Model file for the job. Use its own axes, mm. Face numbers are marked on the shaded views. A direction names the side the tool comes from. Coordinates: 2 decimals unless noted, no trailing zeros. Write each loop counter-clockwise with the first axis right and the second up, starting at its lowest first coordinate (ties: lowest second). Pieces come first, ordered by that corner, then holes.
Q1. Pin check, flat tips, straight feed: P1, Ø0.9, axis at y = 295.5, z = 2, coming from the -X side; P2, Ø1.5, axis at y = 315, z = 1, coming from the +X side; P3, Ø7, axis at y = 453, z = -5, coming from the +X side; P4, Ø3.5, axis at x = 91, z = 2, coming from the +Y side. Stop position of each tip, or through.
Q2. Band-saw the part on A-A, the plane z = -7.5. Write the cut outline in (x, y), plus the area to 3 significant figures.
Q3. Which spindle directions (+Z, -Z, +X, -X, +Y, -Y) get a long thin tool onto all of the face, cutting with end or side? Do the marked faces 1 and 2. Say none if no direction does.
Q4. Band-saw the part on C-C, the plane y = 223. Write the cut outline in (x, z), plus the area to 3 significant figures.
Q5. Drill centre lines: probe 1 along Y at (x, z) = (28, -5); probe 2 along X at (y, z) = (1.85, -15); probe 3 along Y at (x, z) = (-171.5, -24). Where is each one in solid material? Low to high.
Q6. Band-saw the part on B-B, the plane y = 420. Write the cut outline in (x, z).
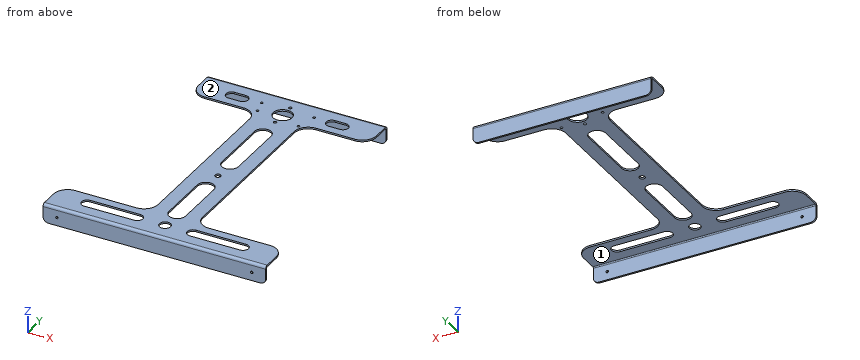
from build123d import *

# Parameters (mm, degrees)
ESQUISSE1_W                             = 400
ESQUISSE1_H                             = 470
BOSS_EXTRU_1_DEPTH                      = 3
T_LE_PLI_E_SUR_AR_TE1_STRIP_W           = 16
T_LE_PLI_E_SUR_AR_TE1_STRIP_H           = 3
T_LE_PLI_E_SUR_AR_TE1_STRIP_CUT_DEPTH   = 400
T_LE_PLI_E_SUR_AR_TE1_STRIP_2_W         = 16
T_LE_PLI_E_SUR_AR_TE1_STRIP_2_H         = 3
T_LE_PLI_E_SUR_AR_TE1_STRIP_CUT_2_DEPTH = 400
T_LE_PLI_E_SUR_AR_TE1_DEPTH             = 400
T_LE_PLI_E_SUR_AR_TE1_BEND_DEPTH        = 400
ENL_V_MAT_EXTRU_1_REACH                 = 513.849
ESQUISSE7_R                             = 17
ESQUISSE7_R_2                           = 5.1
ESQUISSE7_R_3                           = 2.75
ENL_V_MAT_EXTRU_2_REACH                 = 513.849
ESQUISSE12_R                            = 2.25
ESQUISSE12_R_2                          = 10
CONG_10_R                               = 10
CONG_2_R                                = 25
ESQUISSE13_R                            = 2.25
ENL_V_MAT_EXTRU_3_DEPTH                 = 10


# Sheet-metal steps are written as plain solids
with BuildPart() as part:
    # Esquisse1 → Boss.-Extru.1 (new body)
    with BuildSketch(Plane.XY):
        with Locations((0, 235)):
            Rectangle(ESQUISSE1_W, ESQUISSE1_H)
    extrude(amount=BOSS_EXTRU_1_DEPTH)

    # Tôle pliée sur arête1 strip (across the edge) → Tôle pliée sur arête1 strip cut (cut)
    with BuildSketch(Plane(origin=(-200, 470, 0), x_dir=(0, -1, 0), z_dir=(1, 0, 0))):
        with Locations((-3, -1.5)):
            Rectangle(T_LE_PLI_E_SUR_AR_TE1_STRIP_W, T_LE_PLI_E_SUR_AR_TE1_STRIP_H)
    extrude(amount=T_LE_PLI_E_SUR_AR_TE1_STRIP_CUT_DEPTH, mode=Mode.SUBTRACT)

    # Tôle pliée sur arête1 strip 2 (across the edge) → Tôle pliée sur arête1 strip cut 2 (cut)
    with BuildSketch(Plane(origin=(200, 0, 0), x_dir=(0, 1, 0), z_dir=(-1, 0, 0))):
        with Locations((-3, -1.5)):
            Rectangle(T_LE_PLI_E_SUR_AR_TE1_STRIP_2_W, T_LE_PLI_E_SUR_AR_TE1_STRIP_2_H)
    extrude(amount=T_LE_PLI_E_SUR_AR_TE1_STRIP_CUT_2_DEPTH, mode=Mode.SUBTRACT)

    # Tôle pliée sur arête1 section (across the edge) → Tôle pliée sur arête1 (add)
    with BuildSketch(Plane(origin=(-200, 470, 0), x_dir=(0, -1, 0), z_dir=(1, 0, 0))):
        with BuildLine():
            Line((0, 2), (0, 30))
            Line((0, 30), (3, 30))
            Line((3, 30), (3, 2))
            ThreePointArc((3, 2), (3.585786438, 0.585786438), (5, 0))
            Line((5, 0), (5, -3))
            ThreePointArc((5, -3), (1.464466094, -1.535533906), (0, 2))
        make_face()
    extrude(amount=T_LE_PLI_E_SUR_AR_TE1_DEPTH)

    # Tôle pliée sur arête1 section 2 (across the edge) → Tôle pliée sur arête1 bend (add)
    with BuildSketch(Plane(origin=(200, 0, 0), x_dir=(0, 1, 0), z_dir=(-1, 0, 0))):
        with BuildLine():
            Line((0, 2), (0, 30))
            Line((0, 30), (3, 30))
            Line((3, 30), (3, 2))
            ThreePointArc((3, 2), (3.585786438, 0.585786438), (5, 0))
            Line((5, 0), (5, -3))
            ThreePointArc((5, -3), (1.464466094, -1.535533906), (0, 2))
        make_face()
    extrude(amount=T_LE_PLI_E_SUR_AR_TE1_BEND_DEPTH)

    # Esquisse7 → Enlèv. mat.-Extru.1 (cut, up to next)
    with BuildSketch(Plane.XY.offset(3), mode=Mode.PRIVATE) as enl_v_mat_extru_1_sk1:
        with Locations((0, 420)):
            Circle(ESQUISSE7_R)
    enl_v_mat_extru_1_tool1 = extrude(enl_v_mat_extru_1_sk1.sketch, amount=-ENL_V_MAT_EXTRU_1_REACH, mode=Mode.PRIVATE) & part.part
    # Esquisse7 → Enlèv. mat.-Extru.1 (cut, up to next)
    with BuildSketch(Plane.XY.offset(3), mode=Mode.PRIVATE) as enl_v_mat_extru_1_sk2:
        with Locations((0, 208)):
            Circle(ESQUISSE7_R_2)
    enl_v_mat_extru_1_tool2 = extrude(enl_v_mat_extru_1_sk2.sketch, amount=-ENL_V_MAT_EXTRU_1_REACH, mode=Mode.PRIVATE) & part.part
    # Esquisse7 → Enlèv. mat.-Extru.1 (cut, up to next)
    with BuildSketch(Plane.XY.offset(3), mode=Mode.PRIVATE) as enl_v_mat_extru_1_sk3:
        with Locations((0, 395)):
            Circle(ESQUISSE7_R_3)
    enl_v_mat_extru_1_tool3 = extrude(enl_v_mat_extru_1_sk3.sketch, amount=-ENL_V_MAT_EXTRU_1_REACH, mode=Mode.PRIVATE) & part.part
    # Esquisse7 → Enlèv. mat.-Extru.1 (cut, up to next)
    with BuildSketch(Plane.XY.offset(3), mode=Mode.PRIVATE) as enl_v_mat_extru_1_sk4:
        with Locations((0, 445)):
            Circle(ESQUISSE7_R_3)
    enl_v_mat_extru_1_tool4 = extrude(enl_v_mat_extru_1_sk4.sketch, amount=-ENL_V_MAT_EXTRU_1_REACH, mode=Mode.PRIVATE) & part.part
    # Esquisse7 → Enlèv. mat.-Extru.1 (cut, up to next)
    with BuildSketch(Plane.XY.offset(3), mode=Mode.PRIVATE) as enl_v_mat_extru_1_sk5:
        with BuildLine():
            Line((-200, 60), (-65, 60))
            ThreePointArc((-65, 60), (-47.32233047, 67.32233047), (-40, 85))
            Line((-40, 85), (-40, 385))
            ThreePointArc((-40, 385), (-47.32233047, 402.67766953), (-65, 410))
            Line((-65, 410), (-160, 410))
            Line((-160, 410), (-160, 470))
            Line((-160, 470), (-200, 470))
            Line((-200, 470), (-200, 60))
        make_face()
    enl_v_mat_extru_1_tool5 = extrude(enl_v_mat_extru_1_sk5.sketch, amount=-ENL_V_MAT_EXTRU_1_REACH, mode=Mode.PRIVATE) & part.part
    # Esquisse7 → Enlèv. mat.-Extru.1 (cut, up to next)
    with BuildSketch(Plane.XY.offset(3), mode=Mode.PRIVATE) as enl_v_mat_extru_1_sk6:
        with BuildLine():
            Line((200.093993977, 470), (200.093993977, 60))
            Line((200.093993977, 60), (65, 60))
            ThreePointArc((65, 60), (47.32233047, 67.32233047), (40, 85))
            Line((40, 85), (40, 385))
            ThreePointArc((40, 385), (47.32233047, 402.67766953), (65, 410))
            Line((65, 410), (160, 410))
            Line((160, 410), (160, 470))
            Line((160, 470), (200.093993977, 470))
        make_face()
    enl_v_mat_extru_1_tool6 = extrude(enl_v_mat_extru_1_sk6.sketch, amount=-ENL_V_MAT_EXTRU_1_REACH, mode=Mode.PRIVATE) & part.part
    add(enl_v_mat_extru_1_tool1.solids().sort_by_distance((0, 420, 3))[0], mode=Mode.SUBTRACT)
    add(enl_v_mat_extru_1_tool2.solids().sort_by_distance((0, 208, 3))[0], mode=Mode.SUBTRACT)
    add(enl_v_mat_extru_1_tool3.solids().sort_by_distance((0, 395, 3))[0], mode=Mode.SUBTRACT)
    add(enl_v_mat_extru_1_tool4.solids().sort_by_distance((0, 445, 3))[0], mode=Mode.SUBTRACT)
    add(enl_v_mat_extru_1_tool5.solids().sort_by_distance((-122.820528, 243.463534, 3))[0], mode=Mode.SUBTRACT)
    add(enl_v_mat_extru_1_tool6.solids().sort_by_distance((122.87169, 243.477801, 3))[0], mode=Mode.SUBTRACT)

    # Esquisse12 → Enlèv. mat.-Extru.2 (cut, up to next)
    with BuildSketch(Plane.XY.offset(3), mode=Mode.PRIVATE) as enl_v_mat_extru_2_sk1:
        with Locations((38.064927056, 402.250033007)):
            Circle(ESQUISSE12_R)
    enl_v_mat_extru_2_tool1 = extrude(enl_v_mat_extru_2_sk1.sketch, amount=-ENL_V_MAT_EXTRU_2_REACH, mode=Mode.PRIVATE) & part.part
    # Esquisse12 → Enlèv. mat.-Extru.2 (cut, up to next)
    with BuildSketch(Plane.XY.offset(3), mode=Mode.PRIVATE) as enl_v_mat_extru_2_sk2:
        with Locations((-41.361925627, 412.706776538)):
            Circle(ESQUISSE12_R)
    enl_v_mat_extru_2_tool2 = extrude(enl_v_mat_extru_2_sk2.sketch, amount=-ENL_V_MAT_EXTRU_2_REACH, mode=Mode.PRIVATE) & part.part
    # Esquisse12 → Enlèv. mat.-Extru.2 (cut, up to next)
    with BuildSketch(Plane.XY.offset(3), mode=Mode.PRIVATE) as enl_v_mat_extru_2_sk3:
        with Locations((46.984631039, 437.101007166)):
            Circle(ESQUISSE12_R)
    enl_v_mat_extru_2_tool3 = extrude(enl_v_mat_extru_2_sk3.sketch, amount=-ENL_V_MAT_EXTRU_2_REACH, mode=Mode.PRIVATE) & part.part
    # Esquisse12 → Enlèv. mat.-Extru.2 (cut, up to next)
    with BuildSketch(Plane.XY.offset(3), mode=Mode.PRIVATE) as enl_v_mat_extru_2_sk4:
        with Locations((-46.984631039, 437.101007166)):
            Circle(ESQUISSE12_R)
    enl_v_mat_extru_2_tool4 = extrude(enl_v_mat_extru_2_sk4.sketch, amount=-ENL_V_MAT_EXTRU_2_REACH, mode=Mode.PRIVATE) & part.part
    # Esquisse12 → Enlèv. mat.-Extru.2 (cut, up to next)
    with BuildSketch(Plane.XY.offset(3), mode=Mode.PRIVATE) as enl_v_mat_extru_2_sk5:
        with Locations((0, 35)):
            Circle(ESQUISSE12_R_2)
    enl_v_mat_extru_2_tool5 = extrude(enl_v_mat_extru_2_sk5.sketch, amount=-ENL_V_MAT_EXTRU_2_REACH, mode=Mode.PRIVATE) & part.part
    # Esquisse12 → Enlèv. mat.-Extru.2 (cut, up to next)
    with BuildSketch(Plane.XY.offset(3), mode=Mode.PRIVATE) as enl_v_mat_extru_2_sk6:
        with BuildLine():
            Line((-15, 168), (-15, 75))
            ThreePointArc((-15, 75), (0, 60), (15, 75))
            Line((15, 75), (15, 168))
            ThreePointArc((15, 168), (0, 183), (-15, 168))
        make_face()
    enl_v_mat_extru_2_tool6 = extrude(enl_v_mat_extru_2_sk6.sketch, amount=-ENL_V_MAT_EXTRU_2_REACH, mode=Mode.PRIVATE) & part.part
    # Esquisse12 → Enlèv. mat.-Extru.2 (cut, up to next)
    with BuildSketch(Plane.XY.offset(3), mode=Mode.PRIVATE) as enl_v_mat_extru_2_sk7:
        with BuildLine():
            Line((140, 45), (50, 45))
            ThreePointArc((50, 45), (40, 35), (50, 25))
            Line((50, 25), (140, 25))
            ThreePointArc((140, 25), (150, 35), (140, 45))
        make_face()
    enl_v_mat_extru_2_tool7 = extrude(enl_v_mat_extru_2_sk7.sketch, amount=-ENL_V_MAT_EXTRU_2_REACH, mode=Mode.PRIVATE) & part.part
    # Esquisse12 → Enlèv. mat.-Extru.2 (cut, up to next)
    with BuildSketch(Plane.XY.offset(3), mode=Mode.PRIVATE) as enl_v_mat_extru_2_sk8:
        with BuildLine():
            Line((15, 355), (15, 248))
            ThreePointArc((15, 248), (0, 233), (-15, 248))
            Line((-15, 248), (-15, 355))
            ThreePointArc((-15, 355), (0, 370), (15, 355))
        make_face()
    enl_v_mat_extru_2_tool8 = extrude(enl_v_mat_extru_2_sk8.sketch, amount=-ENL_V_MAT_EXTRU_2_REACH, mode=Mode.PRIVATE) & part.part
    # Esquisse12 → Enlèv. mat.-Extru.2 (cut, up to next)
    with BuildSketch(Plane.XY.offset(3), mode=Mode.PRIVATE) as enl_v_mat_extru_2_sk9:
        with BuildLine():
            Line((-140, 45), (-50, 45))
            ThreePointArc((-50, 45), (-40, 35), (-50, 25))
            Line((-50, 25), (-140, 25))
            ThreePointArc((-140, 25), (-150, 35), (-140, 45))
        make_face()
    enl_v_mat_extru_2_tool9 = extrude(enl_v_mat_extru_2_sk9.sketch, amount=-ENL_V_MAT_EXTRU_2_REACH, mode=Mode.PRIVATE) & part.part
    # Esquisse12 → Enlèv. mat.-Extru.2 (cut, up to next)
    with BuildSketch(Plane.XY.offset(3), mode=Mode.PRIVATE) as enl_v_mat_extru_2_sk10:
        with BuildLine():
            Line((-100, 425), (-80, 425))
            ThreePointArc((-80, 425), (-70, 435), (-80, 445))
            Line((-80, 445), (-100, 445))
            ThreePointArc((-100, 445), (-110, 435), (-100, 425))
        make_face()
    enl_v_mat_extru_2_tool10 = extrude(enl_v_mat_extru_2_sk10.sketch, amount=-ENL_V_MAT_EXTRU_2_REACH, mode=Mode.PRIVATE) & part.part
    # Esquisse12 → Enlèv. mat.-Extru.2 (cut, up to next)
    with BuildSketch(Plane.XY.offset(3), mode=Mode.PRIVATE) as enl_v_mat_extru_2_sk11:
        with BuildLine():
            Line((80, 445), (100, 445))
            ThreePointArc((100, 445), (110, 435), (100, 425))
            Line((100, 425), (80, 425))
            ThreePointArc((80, 425), (70, 435), (80, 445))
        make_face()
    enl_v_mat_extru_2_tool11 = extrude(enl_v_mat_extru_2_sk11.sketch, amount=-ENL_V_MAT_EXTRU_2_REACH, mode=Mode.PRIVATE) & part.part
    add(enl_v_mat_extru_2_tool1.solids().sort_by_distance((38.064927, 402.250033, 3))[0], mode=Mode.SUBTRACT)
    add(enl_v_mat_extru_2_tool2.solids().sort_by_distance((-41.361926, 412.706777, 3))[0], mode=Mode.SUBTRACT)
    add(enl_v_mat_extru_2_tool3.solids().sort_by_distance((46.984631, 437.101007, 3))[0], mode=Mode.SUBTRACT)
    add(enl_v_mat_extru_2_tool4.solids().sort_by_distance((-46.984631, 437.101007, 3))[0], mode=Mode.SUBTRACT)
    add(enl_v_mat_extru_2_tool5.solids().sort_by_distance((0, 35, 3))[0], mode=Mode.SUBTRACT)
    add(enl_v_mat_extru_2_tool6.solids().sort_by_distance((0, 121.5, 3))[0], mode=Mode.SUBTRACT)
    add(enl_v_mat_extru_2_tool7.solids().sort_by_distance((95, 35, 3))[0], mode=Mode.SUBTRACT)
    add(enl_v_mat_extru_2_tool8.solids().sort_by_distance((0, 301.5, 3))[0], mode=Mode.SUBTRACT)
    add(enl_v_mat_extru_2_tool9.solids().sort_by_distance((-95, 35, 3))[0], mode=Mode.SUBTRACT)
    add(enl_v_mat_extru_2_tool10.solids().sort_by_distance((-90, 435, 3))[0], mode=Mode.SUBTRACT)
    add(enl_v_mat_extru_2_tool11.solids().sort_by_distance((90, 435, 3))[0], mode=Mode.SUBTRACT)

    # Congé 10
    cong_10_edges = [part.edges().sort_by_distance(p)[0] for p in [
        (160, 468.5, -30),
        (200, 1.5, -30),
        (-200, 1.5, -30),
        (-160, 468.5, -30),
    ]]
    fillet(cong_10_edges, radius=CONG_10_R)

    # Congé2
    cong_2_edges = [part.edges().sort_by_distance(p)[0] for p in [
        (200, 60, 1.5),
        (160, 410, 1.5),
        (-200, 60, 1.5),
        (-160, 410, 1.5),
    ]]
    fillet(cong_2_edges, radius=CONG_2_R)

    # Esquisse13 → Enlèv. mat.-Extru.3 (cut)
    with BuildSketch(Plane(origin=(0, 0, 0), x_dir=(-1, 0, 0), z_dir=(0, -1, 0))):
        with Locations(Location((175, 15, 0), (0, 0, 90))):
            Circle(ESQUISSE13_R)
        with Locations(Location((-175, 15, 0), (0, 0, 90))):
            Circle(ESQUISSE13_R)
    extrude(amount=-ENL_V_MAT_EXTRU_3_DEPTH, mode=Mode.SUBTRACT)


solid = part.part
Answer sheet:
1. P1: stops at x = -40
1. P2: stops at x = 40
1. P3: passes through
1. P4: stops at y = 469.47
2. outline: (-200, 0) - (200, 0) - (200, 3) - (-200, 3) - close; (-160, 467) - (160, 467) - (160, 470) - (-160, 470) - close
2. area: 2,160 mm2
3. face 1: -Z, +X, -X
3. face 2: +Z, +X, -X, +Y, -Y
4. outline: (-40, 0) - (40, 0) - (40, 3) - (-40, 3) - close
4. area: 240 mm2
5. probe 1: y = 0 to 3, 467 to 470
5. probe 2: x = -200 to -177.25, -172.75 to 172.75, 177.25 to 200
5. probe 3: y = 0 to 3
6. outline: (-155, 0) - (-17, 0) - (-17, 3) - (-155, 3) - close; (17, 0) - (155, 0) - (155, 3) - (17, 3) - close
